Autodesk Inventor part; units mm, degrees
ref_plane "YZ Plane" through (0, 0, 0) normal (1, 0, 0) x (0, 1, 0)
ref_plane "XZ Plane" through (0, 0, 0) normal (0, 1, 0) x (-1, 0, 0)
ref_plane "XY Plane" through (0, 0, 0) normal (0, 0, 1) x (1, 0, 0)
sketch "Sketch1" plane through (0, 0, 0) normal (0, 0, 1) x (1, 0, 0)
  circle A0 centre (9.5006, -10.0358) radius 2
  circle A1 centre (-2.9994, -10.0358) radius 2
  circle A2 centre (-2.9994, 10.9642) radius 2
  circle A3 centre (9.5006, 10.9642) radius 2
  line L0 (9.0506, -3.7358) -> (6.9506, -3.7358)
  line L1 (6.9506, -3.7358) -> (-6.3494, -3.7358)
  line L2 (-6.3494, -3.7358) -> (-6.3494, 4.6642)
  line L3 (-6.3494, 4.6642) -> (11.5506, 4.6642)
  line L4 (11.5506, 4.6642) -> (11.5506, -3.7358)
  line L5 (11.5506, -3.7358) -> (9.0506, -3.7358)
  line L6 (9.0506, -3.7358) -> (9.0506, -8.5358) construction
  line L7 (9.0506, -8.5358) -> (6.9506, -8.5358) construction
  line L8 (6.9506, -8.5358) -> (6.9506, -3.7358) construction
  line L9 (-23.9494, 23.9642) -> (-23.9494, -23.0358)
  circle A4 centre (-18.4494, -17.5358) radius 1.4 construction
  circle A5 centre (-18.4494, 18.4642) radius 1.4 construction
  circle A6 centre (17.5506, 18.4642) radius 1.4 construction
  circle A7 centre (17.5506, -17.5358) radius 1.4 construction
  circle A8 centre (-18.4494, -17.5358) radius 1.4 construction
  circle A9 centre (17.5506, -17.5358) radius 1.4 construction
  circle A10 centre (17.5506, 18.4642) radius 1.4 construction
  circle A11 centre (-18.4494, 18.4642) radius 1.4 construction
  circle A12 centre (-2.9994, 10.9642) radius 0.9
  circle A13 centre (9.5006, 10.9642) radius 0.9
  circle A14 centre (9.5006, -10.0358) radius 0.9
  circle A15 centre (-2.9994, -10.0358) radius 0.9
  line L10 (-23.9494, -23.0358) -> (23.0506, -23.0358)
  line L11 (23.0506, -23.0358) -> (23.0506, 23.9642)
  line L12 (23.0506, 23.9642) -> (-23.9494, 23.9642)
  line L13 (10.4426, -23.0358) -> (10.4426, 23.9642) construction
  line L14 (-22.2241, 23.9642) -> (-22.2241, -23.0358) construction
  circle A16 centre (17.5506, -17.5358) radius 2.75
  circle A17 centre (-18.4494, -17.5358) radius 2.75
  circle A18 centre (17.5506, 18.4642) radius 2.75
  circle A19 centre (-18.4494, 18.4642) radius 2.75
  point P0 (0, 0)
extrude "Extrusion1" add sketch "Sketch1" along normal blind 3 contours L12 L11 L10 L9
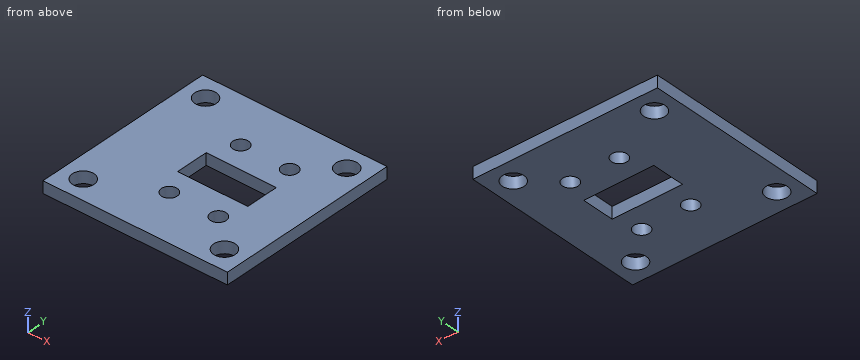
The listing builds one solid part. Answer for the finished solid, in the listing's coordinates (mm). Coordinates: 2 decimals unless noted, no trailing zeros. Loops run counter-clockwise (first coordinate to the right, second up) from the corner with the lowest first, then second, coordinate; pieces in that order, holes last.
1) Find section C-C on y = 17. Write down the section's boundary in (x, z).
2) Find section B-B on z = 1.1. Give the number of separate pieces and of enclosed holes in the cut face, then the cut area to 3 significant figures.
3) Find section D-D on x = -4. Write down the section's boundary in (y, z), then the cut area to 3 significant figures.
4) Find the intervals of material crossed by L1, parallel to Y at x = 16.5, z = 1.4; L2, parallel to X at y = 2, z = 1.05; L3, parallel to X at y = 10.5, z = 1.05, in increasing order.
5) Find section A-A on x = 3. Write down the section's boundary in (y, z).
6) A flat-ended cylindrical pin translates along its axis: pin 1 Ø2.5 at (x, y) = (-3, -10.04) entering from +Z. Find the tip coordinate at first contact, or state that the pin passes through.
Values:
1. outline: (-23.95, 0) - (-20.78, 0) - (-20.78, 3) - (-23.95, 3) - close; (-16.12, 0) - (15.22, 0) - (15.22, 3) - (-16.12, 3) - close; (19.88, 0) - (23.05, 0) - (23.05, 3) - (19.88, 3) - close
2. separate pieces: 1
2. enclosed holes: 9
2. area: 1,910 mm2
3. outline: (-23.04, 0) - (-11.77, 0) - (-11.77, 3) - (-23.04, 3) - close; (-8.3, 0) - (-3.74, 0) - (-3.74, 3) - (-8.3, 3) - close; (4.66, 0) - (9.23, 0) - (9.23, 3) - (4.66, 3) - close; (12.7, 0) - (23.96, 0) - (23.96, 3) - (12.7, 3) - close
3. area: 95.0 mm2
4. L1: y = -23.04 to -20.08, -14.99 to 15.92, 21.01 to 23.96
4. L2: x = -23.95 to -6.35, 11.55 to 23.05
4. L3: x = -23.95 to -4.94, -1.05 to 7.56, 11.45 to 23.05
5. outline: (-23.04, 0) - (-3.74, 0) - (-3.74, 3) - (-23.04, 3) - close; (4.66, 0) - (23.96, 0) - (23.96, 3) - (4.66, 3) - close
6. pin 1: passes through
